```python
from build123d import *
from build123d.topology import SkipClean

# Parameters (mm, degrees)
SKETCH1_W                       = 20
SKETCH1_H                       = 55
BOSS_EXTRUDE1_DEPTH             = 4
CUT_EXTRUDE1_DEPTH              = 30.533878851
CUT_EXTRUDE1_DEPTH_BACK         = 30.533878851
SKETCH2_R                       = 4.075
SKETCH3_R                       = 7.1
SKETCH3_R_2                     = 4.075
BOSS_EXTRUDE2_DEPTH             = 10
BOSS_EXTRUDE2_DIRECTION_2_REACH = 31.534
SKETCH4_W                       = 21
SKETCH4_H                       = 14
BOSS_EXTRUDE3_DEPTH             = 5
CHAMFER1_SIZE                   = 8
CHAMFER1_OF_MIRROR1_SIZE        = 8
FILLET3_R                       = 10
FILLET4_R                       = 5
SKETCH5_R                       = 1.65
CUT_EXTRUDE2_DEPTH              = 36.672993987


with BuildPart() as part:
    # Sketch1 → Boss-Extrude1 (new body)
    with BuildSketch(Plane(origin=(0, 0, 0), x_dir=(1, 0, 0), z_dir=(0, 1, 0))):
        Rectangle(SKETCH1_W, SKETCH1_H)
    extrude(amount=BOSS_EXTRUDE1_DEPTH)

    # Sketch2 → Cut-Extrude1 (cut, two sides: drawn at the far end of the back side and taken through both)
    with BuildSketch(Plane(origin=(0, 4, 0), x_dir=(1, 0, 0), z_dir=(0, 1, 0)).offset(-CUT_EXTRUDE1_DEPTH_BACK)):
        with Locations((0, 25.65)):
            Circle(SKETCH2_R)
    extrude(amount=CUT_EXTRUDE1_DEPTH + CUT_EXTRUDE1_DEPTH_BACK, mode=Mode.SUBTRACT)

    # Sketch3 → Boss-Extrude2 (add)
    with BuildSketch(Plane(origin=(0, 4, 0), x_dir=(1, 0, 0), z_dir=(0, 1, 0))):
        with Locations(Location((0, 25.65, 0), (0, 0, 270))):
            Circle(SKETCH3_R)
        with Locations(Location((0, 25.65, 0), (0, 0, 270))):
            Circle(SKETCH3_R_2, mode=Mode.SUBTRACT)
    extrude(amount=BOSS_EXTRUDE2_DEPTH)

    # Boss-Extrude2 direction 2: up to this face of the body (flat: up to its plane)
    boss_extrude2_direction_2_end = Plane(part.part.faces().sort_by_distance((0, 0, 0.953538914))[0])
    # Sketch3 → Boss-Extrude2 direction 2 (add, up to the picked face)
    with BuildSketch(Plane(origin=(0, 4, 0), x_dir=(1, 0, 0), z_dir=(0, 1, 0)), mode=Mode.PRIVATE) as boss_extrude2_direction_2_sk1:
        with Locations(Location((0, 25.65, 0), (0, 0, 270))):
            Circle(SKETCH3_R)
        with Locations(Location((0, 25.65, 0), (0, 0, 270))):
            Circle(SKETCH3_R_2, mode=Mode.SUBTRACT)
    boss_extrude2_direction_2_tool1 = split(extrude(boss_extrude2_direction_2_sk1.sketch, amount=-BOSS_EXTRUDE2_DIRECTION_2_REACH, mode=Mode.PRIVATE), bisect_by=boss_extrude2_direction_2_end, keep=Keep.BOTH, mode=Mode.PRIVATE)
    add(boss_extrude2_direction_2_tool1.solids().sort_by(Axis((0, 4, -32.549182), (0, -1, 0)))[0])

    # Sketch4 → Boss-Extrude3 (add)
    with BuildSketch(Plane(origin=(10, 0, 0), x_dir=(0, 0, -1), z_dir=(1, 0, 0))):
        with Locations((17, 7)):
            Rectangle(SKETCH4_W, SKETCH4_H)
    boss_extrude3 = extrude(amount=-BOSS_EXTRUDE3_DEPTH)

    # Chamfer1
    chamfer1_edges = [part.edges().sort_by_distance(p)[0] for p in [
        (7.5, 14, -6.5),
    ]]
    chamfer(chamfer1_edges, length=CHAMFER1_SIZE)

    # Mirror1: Boss-Extrude3 across plane
    with SkipClean():  # the faces are left unmerged after this step: merging them gives an invalid solid
        add(boss_extrude3.mirror(Plane(origin=(0, 0, 0), x_dir=(0, 0, 1), z_dir=(1, 0, 0))))

    # Chamfer1 of Mirror1
    chamfer1_of_mirror1_edges = [part.edges().sort_by_distance(p)[0] for p in [
        (-7.5, 14, -6.5),
    ]]
    chamfer(chamfer1_of_mirror1_edges, length=CHAMFER1_OF_MIRROR1_SIZE)

    # Fillet3
    # the kernel refuses this fillet: 10 mm, written as the material it takes off along each edge
    with BuildSketch(Plane(origin=(10, 32.202420855, -27.5), x_dir=(0, 0, 1), z_dir=(0, -1, 0))) as fillet3_piece_1:
        with BuildLine():
            CenterArc((7.280968342, 10), FILLET3_R, 223.272918663, 46.727081337)
            Line((0, 3.145257116), (-0.145619367, 3.008162259))
            ThreePointArc((-0.145619367, 3.008162259), (-0.2, 1.572628558), (-0.2, 0))
            Line((-0.2, 0), (0, -0.2))
            Line((0, -0.2), (7.280968342, -0.2))
            Line((7.280968342, -0.2), (7.280968342, 0))
        make_face()
    extrude(amount=28.202420855, mode=Mode.SUBTRACT)
    with BuildSketch(Plane(origin=(-10, 32.202420855, -27.5), x_dir=(0, 0, 1), z_dir=(0, -1, 0))) as fillet3_piece_2:
        with BuildLine():
            CenterArc((7.280968342, -10), FILLET3_R, 90, 46.727081337)
            Line((0, -3.145257116), (-0.145619367, -3.008162259))
            ThreePointArc((-0.145619367, -3.008162259), (-0.2, -1.572628558), (-0.2, 0))
            Line((-0.2, 0), (0, 0.2))
            Line((0, 0.2), (7.280968342, 0.2))
            Line((7.280968342, 0.2), (7.280968342, 0))
        make_face()
    extrude(amount=28.202420855, mode=Mode.SUBTRACT)
    with BuildSketch(Plane(origin=(-10, -18.202420855, -27.5), x_dir=(0, 0, 1), z_dir=(0, 1, 0))) as fillet3_piece_3:
        with BuildLine():
            CenterArc((7.280968342, 10), FILLET3_R, 223.272918663, 46.727081337)
            Line((0, 3.145257116), (-0.145619367, 3.008162259))
            ThreePointArc((-0.145619367, 3.008162259), (-0.2, 1.572628558), (-0.2, 0))
            Line((-0.2, 0), (0, -0.2))
            Line((0, -0.2), (7.280968342, -0.2))
            Line((7.280968342, -0.2), (7.280968342, 0))
        make_face()
    extrude(amount=22.202420855, mode=Mode.SUBTRACT)
    with BuildSketch(Plane(origin=(10, -18.202420855, -27.5), x_dir=(0, 0, 1), z_dir=(0, 1, 0))) as fillet3_piece_4:
        with BuildLine():
            CenterArc((7.280968342, -10), FILLET3_R, 90, 46.727081337)
            Line((0, -3.145257116), (-0.145619367, -3.008162259))
            ThreePointArc((-0.145619367, -3.008162259), (-0.2, -1.572628558), (-0.2, 0))
            Line((-0.2, 0), (0, 0.2))
            Line((0, 0.2), (7.280968342, 0.2))
            Line((7.280968342, 0.2), (7.280968342, 0))
        make_face()
    extrude(amount=22.202420855, mode=Mode.SUBTRACT)

    # Fillet4
    fillet4_edges = [part.edges().sort_by_distance(p)[0] for p in [
        (10, 2, 27.5),
        (-10, 2, 27.5),
    ]]
    fillet(fillet4_edges, radius=FILLET4_R)

    # Sketch5 → Cut-Extrude2 (cut, through all)
    with BuildSketch(Plane(origin=(0, 4, 0), x_dir=(1, 0, 0), z_dir=(0, 1, 0))):
        with Locations(Location((0, -23.5, 0), (0, 0, 270))):
            Circle(SKETCH5_R)
        with Locations(Location((0, -1.5, 0), (0, 0, 270))):
            Circle(SKETCH5_R)
    extrude(amount=-CUT_EXTRUDE2_DEPTH, mode=Mode.SUBTRACT)


solid = part.part
```
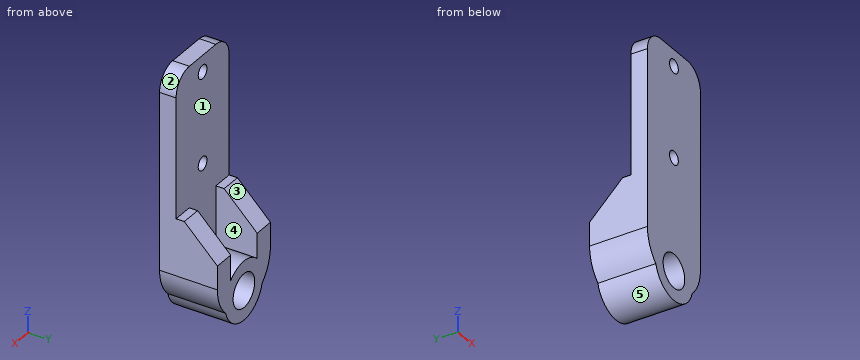
CAD build for the part. Positions are in the model's coordinates, mm. Face numbers are marked on the shaded views. A direction names the side the tool comes from. Coordinates: 2 decimals unless noted, no trailing zeros. Order: outer loops, then holes, each group sorted by start corner. A loop starts at its lowest first (then second) coordinate and runs counter-clockwise, first axis right, second up. Notation, with made-up numbers: (37.5, 11) - (71.5, 11) arc R8 cw to (71.5, 26) - close; hole circle Ø3 at (72.25, 72). An arc over 180 degrees is marked (long way). Use a Markdown table: item, result. Add a question column.
(1) Saw through at B-B (z = 1.5). Give the cut face in (x, y), then the cut area to 3 significant figures.
(2) Drill centre lines: line 1 along X through (y, z) = (6.25, -14); line 2 along Y through (x, z) = (2.5, 8.5); line 3 along Z through (x, y) = (1.75, 5.75). Where is each one in solid material? Low to high. Write a range as [from, to].
(3) Saw through at A-A (x = 0). Give the cut face in (y, z) (3 decimals), then the cut area to 4 significant figures.
(4) Which spindle directions (+Z, -Z, +X, -X, +Y, -Y) get a long thin tool onto all of the face, cutting with end or side? Do the marked faces 4 and 5. Say none if no direction does.
(5) Saw through at C-C (y = 11.25). Give the cut face in (x, z) (3 decimals), then the cut area to 3 significant figures.
(6) Flat gauge pins, fed straight in: pin 1 (0.6 mm diameter, centred on x = 7.5, y = 5.5, fed in from +Z); pin 2 (3 mm diameter, centred on x = 0, z = 1.5, fed in from +Y). Where does each tip first touch, or does it go through?
(7) Pull direction X, two halves, no side cores. Call the marked faces 1, 2 and 3: +X half, -X half, draft (parallel to the pull), parting line (faces both ways), or undercut.
(8) Saw through at D-D (y = 1.25). Give the cut face in (x, z) (3 decimals), then the cut area to 3 significant figures.
Solved:
| question | item | result |
|---|---|---|
| 1 | outline | (-10, 0) - (-1.65, 0) - (-1.65, 4) - (-10, 4) - close; (1.65, 0) - (10, 0) - (10, 4) - (1.65, 4) - close |
| 1 | area | 66.8 mm² |
| 2 | line 1 | x = [-10, -5], [5, 10] |
| 2 | line 2 | y = [0, 4] |
| 2 | line 3 | z = [-32.53, -29.33], [-21.97, -18.77] |
| 3 | outline | (0, -32.75) - (14, -32.75) - (14, -29.725) - (0, -29.725) - close; (0, -21.575) - (14, -21.575) - (14, -18.55) - (4, -18.55) - (4, -0.15) - (0, -0.15) - close; (0, 3.15) - (4, 3.15) - (4, 21.85) - (0, 21.85) - close; (0, 25.15) - (4, 25.15) - (4, 27.5) - (0, 27.5) - close |
| 3 | area | 242.5 mm² |
| 4 | face 4 | +Z, +Y |
| 4 | face 5 | -Z, +Y, -Y |
| 5 | outline | (-10, -20.219) arc R10 ccw to (-6.855, -27.5) arc R7.1 ccw to (6.855, -27.5) arc R10 ccw to (10, -20.219) - (10, -11.75) - (5, -11.75) - (5, -20.609) arc R7.1 ccw to (-5, -20.609) - (-5, -11.75) - (-10, -11.75) - close; hole circle Ø8.15 at (0, -25.65) |
| 5 | area | 227 mm² |
| 6 | pin 1 | stops at z = -6.5 |
| 6 | pin 2 | passes through |
| 7 | face 1 | undercut |
| 7 | face 2 | +X half |
| 7 | face 3 | draft |
| 8 | outline | (-10, -20.219) arc R10 ccw to (-6.855, -27.5) arc R7.1 ccw to (6.855, -27.5) arc R10 ccw to (10, -20.219) - (10, 22.5) arc R5 ccw to (5, 27.5) - (-5, 27.5) arc R5 ccw to (-10, 22.5) - close; hole circle Ø8.15 at (0, -25.65); hole circle Ø3.3 at (0, 1.5); hole circle Ø3.3 at (0, 23.5) |
| 8 | area | 1,060 mm² |
